Source: three-view drawing plus pictorial views. Frame: mm from the lowest corner of the part. A direction names the side the tool comes from. Round coordinates to 2 decimals unless told otherwise and drop trailing zeros. Loops run counter-clockwise (first coordinate to the right, second up) from the corner with the lowest first, then second, coordinate; pieces in that order, holes last. Notation, with made-up numbers: (-24, 65.5) -> (27, 65.5) arc R18 ccw to (27, 89.5) -> close; hole circle Ø11 at (40, -17). An arc over 180 degrees is marked (long way). Return JSON: item names as keys, results as strings. Group by question number.
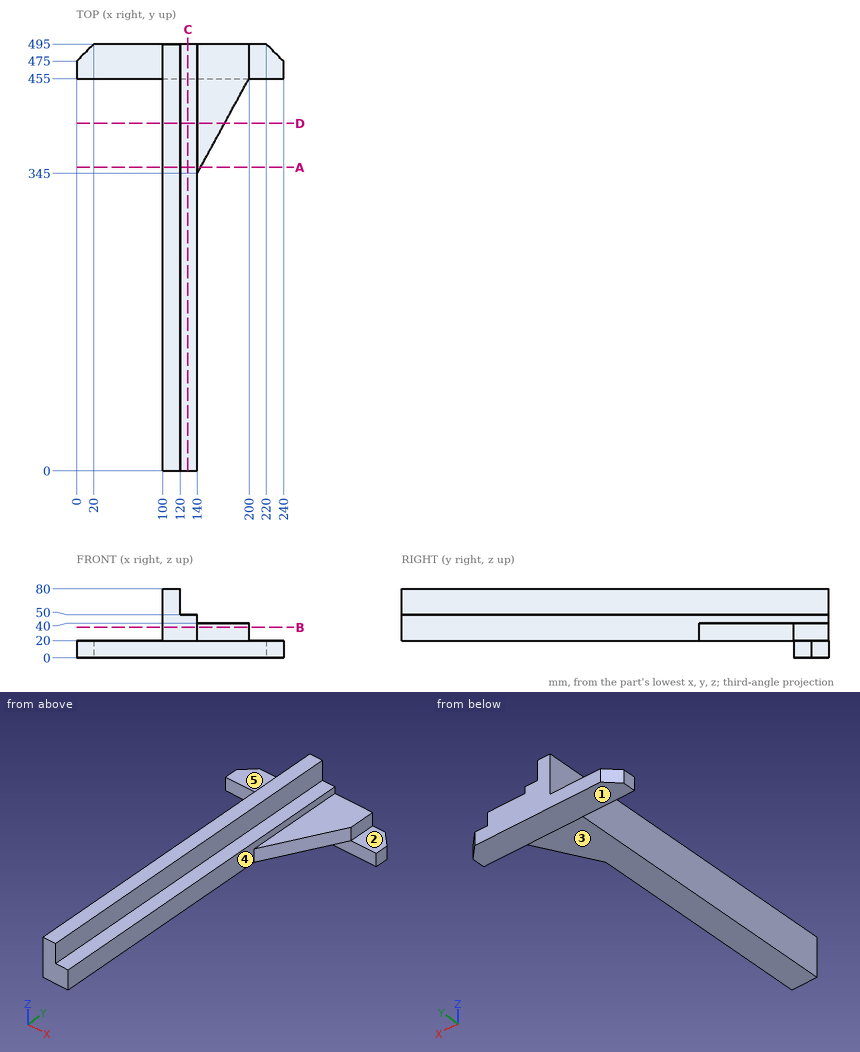
(1) Set-up query: the marked faces 1, 2, 3, 4 and 5. Return all of +Z, -Z, +X, -X, +Y, -Y with unobstructed straight access to the full face (end or side cutting, diameter ignored); none if empty.
(2) Cut plane D-D (y = 403). Return loops of the section in (x, z).
(3) Cut plane B-B (z = 35.5). Return loops of the section in (x, y), and give its area (3 significant figures).
(4) Pin query (flat end, axial travel): pin 1 (18 mm diameter, centred on y = 195.5, z = 48, fed in from -X); pin 2 (10 mm diameter, centred on y = 477, z = 32, fed in from +X); pin 3 (12 mm diameter, centred on y = 63.5, z = 69, fed in from +X); pin 4 (22 mm diameter, centred on x = 125.5, z = 14.5, fed in from -Y). Return the tip coordinate at first contact, or that it passes through.
(5) Ray query, line 1 (Z direction, x = 126, y = 33); line 2 (X direction, y = 400, z = 75.5); line 3 (Y direction, x = 174.5, z = 6). Return the intervals inside material, ascending.
(6) Cut plane C-C (x = 129). Return loops of the section in (y, z), and give its area (4 significant figures).
(7) Cut plane A-A (y = 352). Return loops of the section in (x, z).
Answers follow:
{
 "1": {"face 1": "-Z, +X, -X, +Y, -Y", "face 2": "+Z, +X, +Y, -Y", "face 3": "-Z, +X, -X, -Y", "face 4": "+Z, +X, -Y", "face 5": "+Z, -X, +Y, -Y"},
 "2": {"outline": "(100, 20) -> (171.64, 20) -> (171.64, 40) -> (140, 40) -> (140, 50) -> (120, 50) -> (120, 80) -> (100, 80) -> close"},
 "3": {"outline": "(100, 0) -> (140, 0) -> (140, 345) -> (200, 455) -> (200, 495) -> (100, 495) -> close", "area": "25,500 mm^2"},
 "4": {"pin 1": "x = 100", "pin 2": "x = 200", "pin 3": "x = 120", "pin 4": "y = 0"},
 "5": {"line 1": "20 to 50", "line 2": "100 to 120", "line 3": "455 to 495"},
 "6": {"outline": "(0, 20) -> (455, 20) -> (455, 0) -> (495, 0) -> (495, 50) -> (0, 50) -> close", "area": "15,650 mm^2"},
 "7": {"outline": "(100, 20) -> (143.82, 20) -> (143.82, 40) -> (140, 40) -> (140, 50) -> (120, 50) -> (120, 80) -> (100, 80) -> close"}
}
